Source: three-view drawing plus pictorial views. Frame: mm from the lowest corner of the part. Round coordinates to 2 decimals unless told otherwise and drop trailing zeros. Loops run counter-clockwise (first coordinate to the right, second up) from the corner with the lowest first, then second, coordinate; pieces in that order, holes last. Notation, with made-up numbers: M -29.75,-14.75 L 18.25,-14.75 A27 cw 18.25,10.25 Z; hole C 4.5,2.25 d4. An arc over 180 degrees is marked long. Return JSON: item names as keys, results as strings. Group by question number.
1) Mould query, pull axis X, two halves, no side actions, for the marked faces 1, 2 and 3. Classes: +X half, -X half, draft (parallel to the pull), parting line (faces both ways), or undercut.
2) Contact query for a flat-ended pin moving along its axis: P1, Ø4, axis at x = 4.5, y = 8, coming from the -Z side. Output: stop coordinate, or through.
3) Material intervals for line 1 (Y direction, x = 3, z = 3); line 2 (Y direction, x = 3.5, z = 2); line 3 (X direction, y = 14.5, z = 2.5), sorted ascending. Write a range as from..to.
4) Section A-A (x = 3). Output: boundary loops of the cut face in (y, z), plus the area to 3 significant figures.
5) Section C-C (z = 5.5). Output: boundary loops of the cut face in (x, y), plus the area to 3 significant figures.
6) Section B-B (y = 15). Output: boundary loops of the cut face in (x, z).
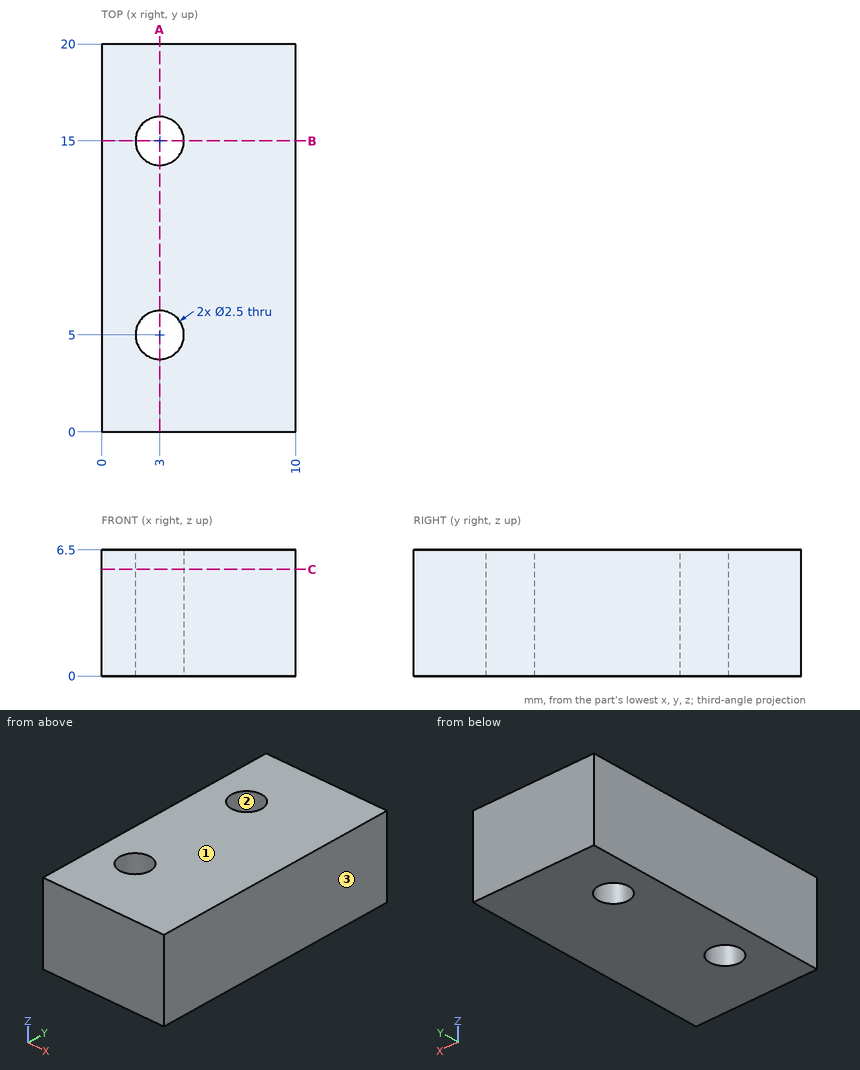
Returned:
{
 "1": {"face 1": "draft", "face 2": "undercut", "face 3": "+X half"},
 "2": {"P1": "stops at z = 0"},
 "3": {"line 1": "y = 0..3.75, 6.25..13.75, 16.25..20", "line 2": "y = 0..3.85, 6.15..13.85, 16.15..20", "line 3": "x = 0..1.85, 4.15..10"},
 "4": {"outline": "M 0,0 L 3.75,0 L 3.75,6.5 L 0,6.5 Z; M 6.25,0 L 13.75,0 L 13.75,6.5 L 6.25,6.5 Z; M 16.25,0 L 20,0 L 20,6.5 L 16.25,6.5 Z", "area": "97.5 mm^2"},
 "5": {"outline": "M 0,0 L 10,0 L 10,20 L 0,20 Z; hole C 3,5 d2.5; hole C 3,15 d2.5", "area": "190 mm^2"},
 "6": {"outline": "M 0,0 L 1.75,0 L 1.75,6.5 L 0,6.5 Z; M 4.25,0 L 10,0 L 10,6.5 L 4.25,6.5 Z"}
}
